Read the model definition and answer for the solid it produces. Units are mm, in the model's axes. Coordinates: 2 decimals unless noted, no trailing zeros. Loops run counter-clockwise (first coordinate to the right, second up) from the corner with the lowest first, then second, coordinate; pieces in that order, holes last.
from build123d import *

# Parameters (mm, degrees)
SKETCH1_R           = 3
BOSS_EXTRUDE1_DEPTH = 95
CHAMFER1_SIZE       = 0.5
CHAMFER1_SIZE2      = 2
CHAMFER2_SIZE       = 2
CHAMFER2_SIZE2      = 0.5
SKETCH2_W           = 6
SKETCH2_H           = 5
CUT_EXTRUDE1_DEPTH  = 0.5


with BuildPart() as part:
    # Sketch1 → Boss-Extrude1 (new body)
    with BuildSketch(Plane(origin=(0, 0, 0), x_dir=(1, 0, 0), z_dir=(0, 1, 0))):
        with Locations(Location((0, 0, 0), (0, 0, 270))):
            Circle(SKETCH1_R)
    extrude(amount=BOSS_EXTRUDE1_DEPTH)

    # Chamfer1
    chamfer1_edges = [part.edges().sort_by_distance(p)[0] for p in [
        (0, 0, -3),
    ]]
    chamfer1_side = [part.faces().sort_by_distance(p)[0] for p in [
        (0, 0, 0),
    ]]
    chamfer(chamfer1_edges, length=CHAMFER1_SIZE, length2=CHAMFER1_SIZE2, reference=chamfer1_side[0])

    # Chamfer2
    chamfer2_edges = [part.edges().sort_by_distance(p)[0] for p in [
        (0, 95, -3),
    ]]
    chamfer2_side = [part.faces().sort_by_distance(p)[0] for p in [
        (0, 48.5, -3),
    ]]
    chamfer(chamfer2_edges, length=CHAMFER2_SIZE, length2=CHAMFER2_SIZE2, reference=chamfer2_side[0])

    # Sketch2 → Cut-Extrude1 (cut)
    with BuildSketch(Plane(origin=(3, 0, 0), x_dir=(0, 0, -1), z_dir=(1, 0, 0))):
        with Locations((0, 16)):
            Rectangle(SKETCH2_W, SKETCH2_H)
    extrude(amount=-CUT_EXTRUDE1_DEPTH, mode=Mode.SUBTRACT)


solid = part.part
Q1. A flat-ended cylindrical pin translates along its axis: pin 1 Ø1.7 at (y, z) = (17, 0.5) entering from +X. Find the tip coordinate at first contact, or state that the pin passes through.
Findings below:
pin 1: stops at x = 2.5
Q2. Straight lines are drawn through the part: probe 1 along Z at (x, y) = (-0.1, 12); probe 2 along Z at (x, y) = (-2.35, 63). For each, find the intervals that lie inside material, in ascending order.
Findings below:
probe 1: z = -3 to 3
probe 2: z = -1.86 to 1.86
Q3. Determine the mould class of faces 1 (the face through (2.5, 16, 0)), 2 (the face through (0.775, 94.681, 2.461)), 3 (the face through (-2.93, 46.86, -0.65)) for opening direction Y: +Y half, -Y half, draft (parallel to the pull), parting line (faces both ways), or undercut.
Findings below:
face 1: undercut
face 2: +Y half
face 3: draft
Q4. A cutting plane is placed at A-A (y = 11.5). Give the vertices of the cut face in (x, z), then the cut area to 3 significant figures.
Findings below:
outline: circle Ø6 at (0, 0)
area: 28.3 mm2
